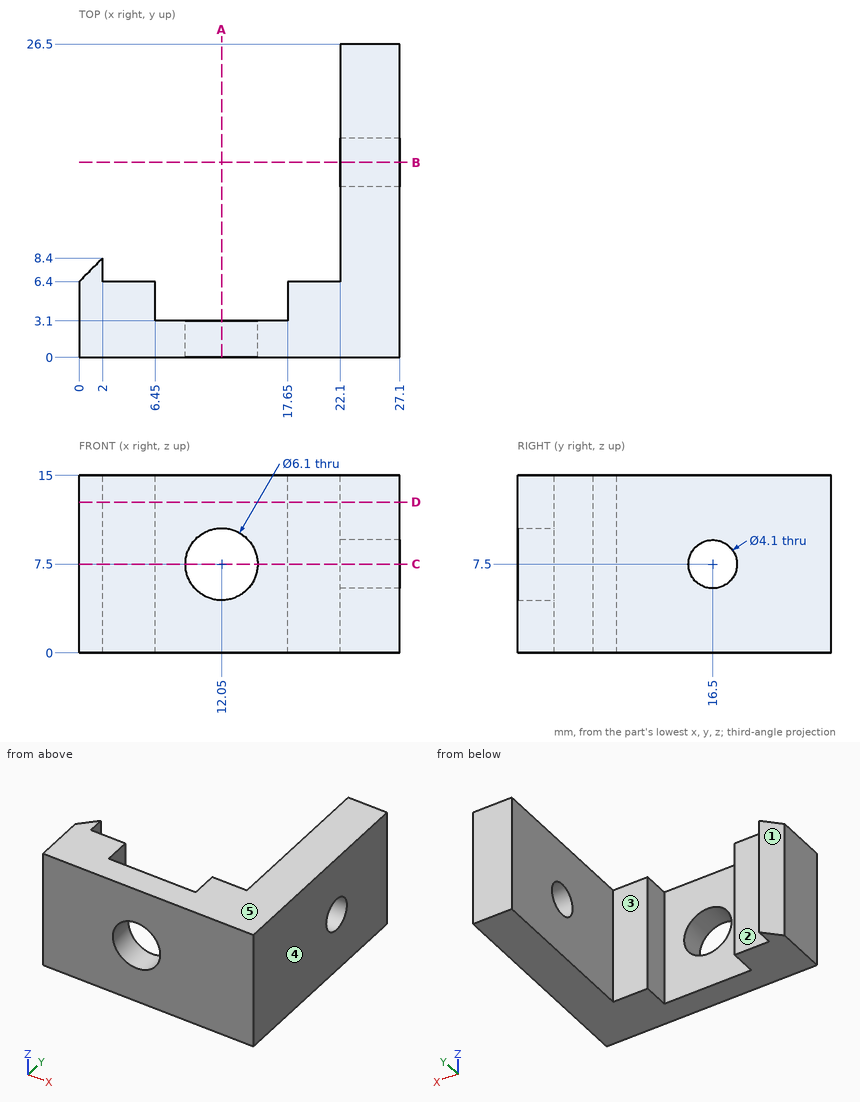
Here's the drawing with two shaded views (mm, measured from the low corner). I have some questions. A direction names the side the tool comes from. Coordinates: 2 decimals unless noted, no trailing zeros. Write each loop counter-clockwise with the first axis right and the second up, starting at its lowest first coordinate (ties: lowest second). Pieces come first, ordered by that corner, then holes. Notation, with made-up numbers: M 26,-27 L 31,-27 A23 cw 31,-12 Z; hole C 27.25,78 d5. An arc over 180 degrees is marked long. Use one line per item in the form item = value.
Q1. We'd pull the mould along X, two halves only. Please class the marked faces 3, 4 and 5: +X half, -X half, draft (parallel to the pull), parting line (faces both ways), or undercut.
Model answer:
face_3 = undercut
face_4 = +X half
face_5 = draft
Q2. For the marked faces 1 and 2, which set-ups out of +Z, -Z, +X, -X, +Y, -Y let a thin tool reach every point of the face, with its end or its side?
Model answer:
face_1 = +Z, -Z, -X, +Y
face_2 = +Z, -Z, +Y
Q3. I need wall thicknesses on line 1 along Z through (x, y) = (12.05, 1.8); line 2 along Z through (x, y) = (25.2, 16.5); line 3 along X through (y, z) = (24.5, 12.75). Which ranges of each line are inside material? Lowest first, please. Write a range as from..to.
Model answer:
line_1 = 0..4.45, 10.55..15
line_2 = 0..5.45, 9.55..15
line_3 = 22.1..27.1
Q4. For P1, Ø4.5, axis at y = 15.5, z = 10, coming from the -X side; P2, Ø4, axis at x = 20, z = 9, coming from the +Y side; P3, Ø5.5, axis at x = 12.05, z = 7.5, coming from the +Y side, each with a flat end and sliding along its axis, tell me the tip position at first contact or that it passes through.
Model answer:
P1 = 22.1
P2 = 6.4
P3 = through
Q5. If we section it at A-A (x = 12.05): Write out the boundary of the cut face in (y, z).
Model answer:
outline = M 0,0 L 3.1,0 L 3.1,4.45 L 0,4.45 Z; M 0,10.55 L 3.1,10.55 L 3.1,15 L 0,15 Z
Q6. If we section it at C-C (z = 7.5): Write out the boundary of the cut face in (x, y).
Model answer:
outline = M 0,0 L 9,0 L 9,3.1 L 6.45,3.1 L 6.45,6.4 L 2,6.4 L 2,8.4 L 0,6.4 Z; M 15.1,0 L 27.1,0 L 27.1,14.45 L 22.1,14.45 L 22.1,6.4 L 17.65,6.4 L 17.65,3.1 L 15.1,3.1 Z; M 22.1,18.55 L 27.1,18.55 L 27.1,26.5 L 22.1,26.5 Z
Q7. If we section it at B-B (y = 16.5): Write out the boundary of the cut face in (x, z).
Model answer:
outline = M 22.1,0 L 27.1,0 L 27.1,5.45 L 22.1,5.45 Z; M 22.1,9.55 L 27.1,9.55 L 27.1,15 L 22.1,15 Z
Q8. If we section it at D-D (z = 12.75): Write out the boundary of the cut face in (x, y).
Model answer:
outline = M 0,0 L 27.1,0 L 27.1,26.5 L 22.1,26.5 L 22.1,6.4 L 17.65,6.4 L 17.65,3.1 L 6.45,3.1 L 6.45,6.4 L 2,6.4 L 2,8.4 L 0,6.4 Z
